```python
from build123d import *

# Parameters (mm, degrees)
F1_DEPTH = 10


with BuildPart() as f1:
    # F0 (on Top) → F1 (new body)
    with BuildSketch(Plane.XY):
        Polygon((0, 43.3012701892), (-75, 43.3012701892), (-37.5, -21.6506350946), (-31.7264973081, -11.6506350946), (-57.6794919243, 33.3012701892), (-5.7735026919, 33.3012701892), align=None)
        Polygon((5.7735026919, 33.3012701892), (-5.7735026919, 33.3012701892), (-31.7264973081, -11.6506350946), (-28.8397459622, -16.6506350946), (-20.1794919243, -11.6506350946), (0, 23.3012701892), (10.0897459622, 5.8253175473), (18.75, 10.8253175473), align=None)
        Polygon((5.7735026919, 33.3012701892), (0, 43.3012701892), (-5.7735026919, 33.3012701892), align=None)
        Polygon((75, 43.3012701892), (0, 43.3012701892), (5.7735026919, 33.3012701892), (57.6794919243, 33.3012701892), align=None)
        Polygon((-20.1794919243, -11.6506350946), (-28.8397459622, -16.6506350946), (-25.9529946162, -21.6506350946), (25.9529946162, -21.6506350946), (31.7264973081, -11.6506350946), (18.75, 10.8253175473), (10.0897459622, 5.8253175473), (20.1794919243, -11.6506350946), align=None)
        Polygon((37.5, -21.6506350946), (75, 43.3012701892), (57.6794919243, 33.3012701892), (31.7264973081, -11.6506350946), align=None)
        Polygon((25.9529946162, -21.6506350946), (37.5, -21.6506350946), (31.7264973081, -11.6506350946), align=None)
        Polygon((-25.9529946162, -21.6506350946), (-37.5, -21.6506350946), (0, -86.6025403784), (37.5, -21.6506350946), (25.9529946162, -21.6506350946), (0, -66.6025403784), align=None)
        Polygon((-31.7264973081, -11.6506350946), (-37.5, -21.6506350946), (-28.8397459622, -16.6506350946), align=None)
        Polygon((-28.8397459622, -16.6506350946), (-37.5, -21.6506350946), (-25.9529946162, -21.6506350946), align=None)
    extrude(amount=F1_DEPTH)


solid = f1.part
```
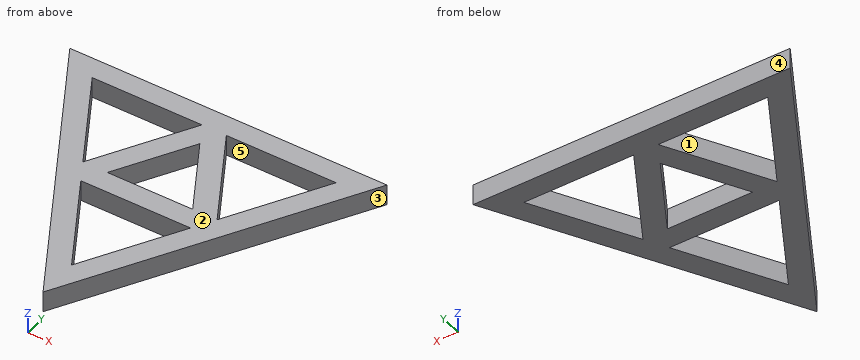
Check sheet for the modelled part. Datum: model origin and axes. Units: mm. Face numbers are marked on the shaded views. A direction names the side the tool comes from. Round coordinates to 2 decimals unless told otherwise and drop trailing zeros. Write each loop counter-clockwise with the first axis right and the second up, starting at its lowest first coordinate (ties: lowest second). Pieces come first, ordered by that corner, then holes. Notation, with made-up numbers: M -33,36 L -11,36 A17 ccw -11,40 Z; hole C -32.75,-18.75 d8. An arc over 180 degrees is marked long. Write item = value, one per line. Start each with the question number.
1. Section check D-D, the plane x = -33.5. Record the cut outline in (y, z), then the cut area to 3 significant figures.
2. Tool access check on the marked faces 4 and 5. Record the directions out of +Z, -Z, +X, -X, +Y, -Y that give a thin tool (end or side, any length) a straight path to the whole face; none if there is none.
3. Release check for a two-part mould opening along X. For the marked faces 1, 2 and 3 record: pulls with the +X half, pulls with the -X half, needs draft (parallel to the pull), parting line crosses it, or undercut.
4. Scan lines: line 1 (Y direction, x = 23.5, z = 8.25); line 2 (Y direction, x = -25, z = 8.5); line 3 (Y direction, x = 11.5, z = 3.75). Record each from-to range of solid material in increasing order. Write a range as [from, to].
5. Section check C-C, the plane y = -35. Record the cut outline in (x, z).
6. Section check B-B, the plane x = 15.5. Record the cut outline in (y, z), then the cut area to 3 significant figures.
7. Section check A-A, the plane z = 3.5. Record the cut outline in (x, y).
8. Gauge pin test, flat ends, axial feed: pin 1 (1 mm diameter, centred on y = -31, z = 7.5, fed in from +X); pin 2 (5 mm diameter, centred on x = 2, z = 4, fed in from -Y); pin 3 (1 mm diameter, centred on y = -65.5, z = 2, fed in from -X). Record the tip position at first contact, or that the pin passes through.
Results found:
q1.outline = M -28.58,0 L -8.58,0 L -8.58,10 L -28.58,10 Z; M 33.3,0 L 43.3,0 L 43.3,10 L 33.3,10 Z
q1.area = 300 mm^2
q2.face_4 = +Z, -Z, +X, -X, +Y
q2.face_5 = +Z, -Z
q3.face_1 = undercut
q3.face_2 = needs draft
q3.face_3 = pulls with the +X half
q4.line_1 = [-45.9, -25.9], [-21.65, 2.6], [33.3, 43.3]
q4.line_2 = [-43.3, -23.3], [-21.65, 0], [33.3, 43.3]
q4.line_3 = [-66.68, -46.68], [-21.65, -11.65], [3.38, 23.38], [33.3, 43.3]
q5.outline = M -29.79,0 L -18.25,0 L -18.25,10 L -29.79,10 Z; M 18.25,0 L 29.79,0 L 29.79,10 L 18.25,10 Z
q6.outline = M -59.76,0 L -39.76,0 L -39.76,10 L -59.76,10 Z; M -21.65,0 L -11.65,0 L -11.65,10 L -21.65,10 Z; M -3.55,0 L 16.45,0 L 16.45,10 L -3.55,10 Z; M 33.3,0 L 43.3,0 L 43.3,10 L 33.3,10 Z
q6.area = 600 mm^2
q7.outline = M -75,43.3 L 0,-86.6 L 75,43.3 Z; hole M -57.68,33.3 L -31.73,-11.65 L -5.77,33.3 Z; hole M -25.95,-21.65 L 0,-66.6 L 25.95,-21.65 Z; hole M -20.18,-11.65 L 20.18,-11.65 L 0,23.3 Z; hole M 5.77,33.3 L 31.73,-11.65 L 57.68,33.3 Z
q8.pin_1 = 32.39
q8.pin_2 = -86.6
q8.pin_3 = -12.47
